Design review of the part shown in the three views and the two pictorial views. Dimensions are in mm from the part's minimum x, y and z. A direction names the side the tool comes from. Coordinates: 2 decimals unless noted, no trailing zeros. Order: outer loops, then holes, each group sorted by start corner. A loop starts at its lowest first (then second) coordinate and runs counter-clockwise, first axis right, second up. Notation, with made-up numbers: (65.25, 21) - (92.25, 21) arc R23 cw to (92.25, 56) - close; hole circle Ø7 at (-31.5, 48). An arc over 180 degrees is marked (long way). One line per item, written item: value. Start each with the question number.
(1) Consider section A-A on x = 19.07. Write out the cut boundary in (y, z).
(2) Clearance check with flat-ended pins moving along their axes: pin 1 (5 mm diameter, centred on y = 16, z = 25, fed in from -X); pin 2 (3 mm diameter, centred on y = 17.5, z = 8.5, fed in from +X); pin 3 (6 mm diameter, centred on x = 31.5, y = 11, fed in from +Z) (1 decimal). State where each tip first meets the part, or that it passes through.
(3) Consider section B-B on y = 25.5. Write out the cut boundary in (x, z), then the cut area to 3 significant figures.
(4) For the marked faces 4 and 5, list the 3-axis set-ups (+Z, -Z, +X, -X, +Y, -Y) from which the entire face can be reached by the end or side of a thin tool; tool diameter is ignored.
(5) Mouldability with a two-part tool opening along Z and no side actions: class the marked faces 1, 2 and 3 as released by +Z, released by -Z, zero draft, split by the parting line, or undercut.
(6) Consider section C-C on z = 24. Write out the cut boundary in (x, y).
(7) Consider section D-D on z = 31. Write out the cut boundary in (x, y).
(8) To check wall thickness, follow line 1 along Y through (x, z) = (12, 36.5); line 2 along X through (y, z) = (7, 15); line 3 along Z through (x, y) = (18.5, 14). State the ranges of each line that lie inside material, in increasing order.
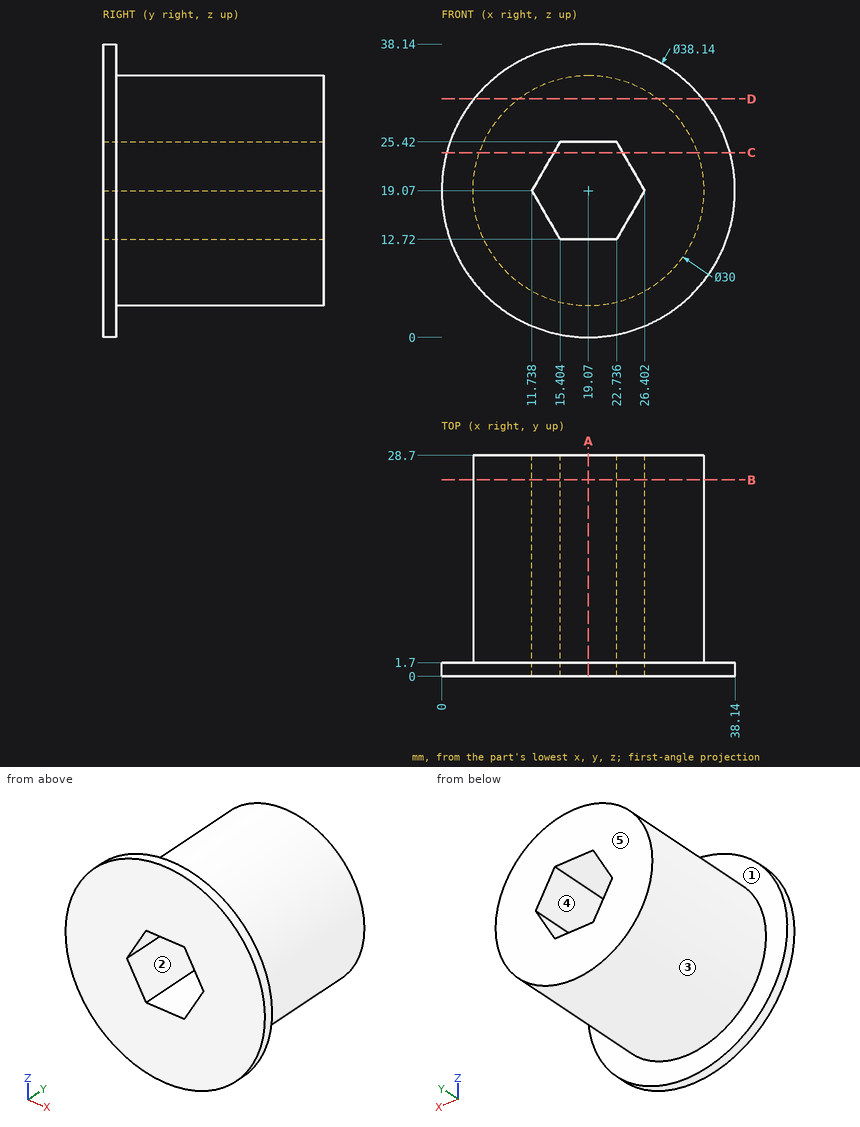
Geometry check:
1. outline: (0, 0) - (1.7, 0) - (1.7, 4.07) - (28.7, 4.07) - (28.7, 12.72) - (0, 12.72) - close; (0, 25.42) - (28.7, 25.42) - (28.7, 34.07) - (1.7, 34.07) - (1.7, 38.14) - (0, 38.14) - close
2. pin 1: stops at x = 4.47
2. pin 2: stops at x = 31.02
2. pin 3: stops at z = 30.7
3. outline: circle Ø30 at (19.07, 19.07); hole (11.74, 19.07) - (15.4, 12.72) - (22.74, 12.72) - (26.4, 19.07) - (22.74, 25.42) - (15.4, 25.42) - close
3. area: 567 mm^2
4. face 4: +Y, -Y
4. face 5: +Z, -Z, +X, -X, +Y
5. face 1: zero draft
5. face 2: undercut
5. face 3: split by the parting line
6. outline: (0.65, 0) - (14.58, 0) - (14.58, 28.7) - (4.9, 28.7) - (4.9, 1.7) - (0.65, 1.7) - close; (23.56, 0) - (37.49, 0) - (37.49, 1.7) - (33.24, 1.7) - (33.24, 28.7) - (23.56, 28.7) - close
7. outline: (4.19, 0) - (33.95, 0) - (33.95, 1.7) - (28.16, 1.7) - (28.16, 28.7) - (9.98, 28.7) - (9.98, 1.7) - (4.19, 1.7) - close
8. line 1: y = 0 to 1.7
8. line 2: x = 4.63 to 14.09, 24.05 to 33.51
8. line 3: z = 4.08 to 12.72, 25.42 to 34.06
